```python
from build123d import *

# Parameters (mm, degrees)
SKETCH2_R           = 5
BOSS_EXTRUDE1_DEPTH = 10
SKETCH3_R           = 10
SKETCH3_R_2         = 5
BOSS_EXTRUDE2_DEPTH = 76.2
BOSS_EXTRUDE3_START = 86.2
SKETCH2_2_R         = 5
BOSS_EXTRUDE3_DEPTH = 22
SKETCH5_R           = 65
BOSS_EXTRUDE4_DEPTH = 22
SKETCH6_R           = 55
CUT_EXTRUDE1_DEPTH  = 22
SKETCH7_R           = 80
CUT_EXTRUDE2_DEPTH  = 22
SKETCH8_R           = 80
CUT_EXTRUDE3_DEPTH  = 10


with BuildPart() as part:
    # Sketch2 → Boss-Extrude1 (new body)
    with BuildSketch(Plane.XY):
        with BuildLine():
            Line((-19.794866372, 2.857142857), (-9.897433186, 71.428571429))
            ThreePointArc((-9.897433186, 71.428571429), (0, 80), (9.897433186, 71.428571429))
            Line((9.897433186, 71.428571429), (19.794866372, 2.857142857))
            ThreePointArc((19.794866372, 2.857142857), (0, -20), (-19.794866372, 2.857142857))
        make_face()
        with Locations((0, 70)):
            Circle(SKETCH2_R, mode=Mode.SUBTRACT)
        with BuildLine():
            Line((-2.5, 9.682458366), (-2.5, 12))
            Line((-2.5, 12), (2.5, 12))
            Line((2.5, 12), (2.5, 9.682458366))
            ThreePointArc((2.5, 9.682458366), (0, -10), (-2.5, 9.682458366))
        make_face(mode=Mode.SUBTRACT)
    extrude(amount=BOSS_EXTRUDE1_DEPTH)

    # Sketch3 → Boss-Extrude2 (add)
    with BuildSketch(Plane.XY.offset(10)):
        with Locations(Location((0, 70, 0), (0, 0, 171.786789298))):
            Circle(SKETCH3_R)
        with Locations((0, 70)):
            Circle(SKETCH3_R_2, mode=Mode.SUBTRACT)
    extrude(amount=BOSS_EXTRUDE2_DEPTH)

    # Sketch2<2> → Boss-Extrude3 (add)
    with BuildSketch(Plane.XY.offset(BOSS_EXTRUDE3_START)):
        with BuildLine():
            Line((-19.794866372, 2.857142857), (-9.897433186, 71.428571429))
            ThreePointArc((-9.897433186, 71.428571429), (0, 80), (9.897433186, 71.428571429))
            Line((9.897433186, 71.428571429), (19.794866372, 2.857142857))
            ThreePointArc((19.794866372, 2.857142857), (0, -20), (-19.794866372, 2.857142857))
        make_face()
        with Locations((0, 70)):
            Circle(SKETCH2_2_R, mode=Mode.SUBTRACT)
        with BuildLine():
            Line((-2.5, 9.682458366), (-2.5, 12))
            Line((-2.5, 12), (2.5, 12))
            Line((2.5, 12), (2.5, 9.682458366))
            ThreePointArc((2.5, 9.682458366), (0, -10), (-2.5, 9.682458366))
        make_face(mode=Mode.SUBTRACT)
    extrude(amount=BOSS_EXTRUDE3_DEPTH)

    # Sketch5 → Boss-Extrude4 (add)
    with BuildSketch(Plane.XY.offset(108.2)):
        Circle(SKETCH5_R)
    extrude(amount=-BOSS_EXTRUDE4_DEPTH)

    # Sketch6 → Cut-Extrude1 (cut)
    with BuildSketch(Plane.XY.offset(108.2)):
        Circle(SKETCH6_R)
    extrude(amount=-CUT_EXTRUDE1_DEPTH, mode=Mode.SUBTRACT)

    # Sketch7 → Cut-Extrude2 (cut)
    with BuildSketch(Plane.XY.offset(108.2)):
        Circle(SKETCH7_R)
    extrude(amount=-CUT_EXTRUDE2_DEPTH, mode=Mode.SUBTRACT)

    # Sketch8 → Cut-Extrude3 (cut)
    with BuildSketch(Plane(origin=(0, 0, 0), x_dir=(-1, 0, 0), z_dir=(0, 0, -1))):
        Circle(SKETCH8_R)
    extrude(amount=-CUT_EXTRUDE3_DEPTH, mode=Mode.SUBTRACT)


solid = part.part
```
For this review, take the finished solid that the model builds, in its own axes (mm). Round coordinates to 2 decimals unless told otherwise and drop trailing zeros. Write each loop counter-clockwise with the first axis right and the second up, starting at its lowest first coordinate (ties: lowest second). Pieces come first, ordered by that corner, then holes.
1) Take a section at A-A on y = 70. Give the boundary of the cut face in (x, z).
Answer below:
outline: (-10, 10) - (-5, 10) - (-5, 86.2) - (-10, 86.2) - close; (5, 10) - (10, 10) - (10, 86.2) - (5, 86.2) - close
2) Insertion check: pin 1 Ø5 at (x, z) = (4, 20) entering from -Y; pin 2 Ø2 at (x, z) = (6.5, 68) entering from -Y; pin 3 Ø6 at (y, z) = (62, 59.5) entering from +X. Each pin has a flat end and moves straight along its axis. Give the tip position at first contact, or say it passes through.
Answer below:
pin 1: stops at y = 60.11
pin 2: stops at y = 61.65
pin 3: stops at x = 8.66
3) Take a section at C-C on z = 15. Give the boundary of the cut face in (x, y), then the cut area to 3 significant figures.
Answer below:
outline: circle Ø20 at (0, 70); hole circle Ø10 at (0, 70)
area: 236 mm2
4) Mouldability with a two-part tool opening along Y and no side actions: class faces 1 (the face through (-8.6, 75.1, 47.6)), 2 (the face through (5, 68, 10)), 3 (the face through (-1.08, 65.12, 47.57)) as +Y half, -Y half, draft (parallel to the pull), parting line (faces both ways), or undercut.
Answer below:
face 1: parting line
face 2: draft
face 3: undercut
5) Take a section at D-D on y = 63. Give the boundary of the cut face in (x, z).
Answer below:
outline: (-7.14, 10) - (7.14, 10) - (7.14, 86.2) - (-7.14, 86.2) - close
6) For line 1 along Y through (x, z) = (0, 60); line 2 along X through (y, z) = (70, 54); line 3 along X through (y, z) = (72.75, 29), list the stretches that pass through material, from the lowest coordinate up.
Answer below:
line 1: y = 60 to 65, 75 to 80
line 2: x = -10 to -5, 5 to 10
line 3: x = -9.61 to -4.18, 4.18 to 9.61
7) Take a section at B-B on x = 0.5. Give the boundary of the cut face in (y, z), then the cut area to 3 significant figures.
Answer below:
outline: (60.01, 10) - (65.03, 10) - (65.03, 86.2) - (60.01, 86.2) - close; (74.97, 10) - (79.99, 10) - (79.99, 86.2) - (74.97, 86.2) - close
area: 764 mm2
